Verification items for the finished model (mm, model axes). Face numbers are marked on the shaded views. A direction names the side the tool comes from. Round coordinates to 2 decimals unless told otherwise and drop trailing zeros. Write each loop counter-clockwise with the first axis right and the second up, starting at its lowest first coordinate (ties: lowest second). Pieces come first, ordered by that corner, then holes. Notation, with made-up numbers: (23, -27.5) - (62, -27.5) arc R26 ccw to (62, -13.5) - close; hole circle Ø2 at (60.5, 74.25). An arc over 180 degrees is marked (long way). Answer as a JSON object with one key per item and string values.
Autodesk Inventor part; units mm, degrees
ref_plane "YZ Plane" through (0, 0, 0) normal (1, 0, 0) x (0, 1, 0)
ref_plane "XZ Plane" through (0, 0, 0) normal (0, 1, 0) x (-1, 0, 0)
ref_plane "XY Plane" through (0, 0, 0) normal (0, 0, 1) x (1, 0, 0)
sketch "Skizze1" plane through (0, 0, 0) normal (0, 0, 1) x (1, 0, 0)
  line L0 (0, 0) -> (12, 0)
  line L1 (12, 0) -> (12, 12)
  line L2 (12, 12) -> (0, 12)
  line L3 (0, 12) -> (0, 0)
  dimension "d0" = 12
  dimension "d1" = 12
extrude "Extrusion1" add sketch "Skizze1" along normal blind 5
sketch "Skizze2" plane through (0, 0, 5) normal (0, 0, 1) x (1, 0, 0)
  circle A0 centre (6, 6) radius 1
  line L0 (12, 0) -> (12, 12)
  line L1 (0, 0) -> (12, 0)
  dimension "d4" = 6
  dimension "d5" = 6
  dimension "d6" = 2
extrude "Extrusion2" add sketch "Skizze2" along normal blind 3
chamfer "Fase1" distance 0.5 angle 45 1 edges at (5, 6, 8)
sketch "Skizze3" plane through (0, 12, 0) normal (0, 1, 0) x (1, 0, 0)
  line L0 (0, 0) -> (12, 0)
  circle A0 centre (6, 0) radius 2.25
  dimension "d12" = 4.5
extrude "Extrusion3" cut sketch "Skizze3" against normal blind 4
sketch "Skizze4" plane through (0, 0, 0) normal (0, 0, -1) x (-1, 0, 0)
  circle A0 centre (-6, 6) radius 0.5
  circle A1 centre (-6, 6) radius 5.4
  point P0 (0, 0)
ref_plane "Arbeitsebene1" through (0, 0, 0.5) normal (0, 0, -1) x (-1, 0, 0)
sketch "Skizze5" plane through (0, 0, 0.5) normal (0, 0, -1) x (-1, 0, 0)
  circle A0 centre (-6, 6) radius 0.5
  circle A1 centre (-6, 6) radius 3.55
  point P0 (0, 0)
  dimension "d18" = 7.1
extrude "Extrusion5" cut sketch "Skizze5" against normal blind 2.7
sketch "Skizze6" plane through (0, 12, 5) normal (0, 1, 0) x (1, 0, 0)
  line L0 (12, 4.5) -> (0, 4.5)
  line L1 (0, 4.5) -> (0, 5)
  line L2 (0, 5) -> (12, 5)
  line L3 (12, 5) -> (12, 4.5)
  line L4 (0, 5) -> (0, 0)
  line L5 (3.75, 5) -> (0, 5)
  line L6 (12, 5) -> (12, 0)
  line L7 (3.8063, 4.5) -> (8.1937, 4.5)
  dimension "d24" = 0
  dimension "d25" = 0
  dimension "d26" = 0
  dimension "d27" = 0
extrude "Extrusion6" cut sketch "Skizze6" against normal blind 20
fillet "Rundung1" radius 2 1 edges at (9.55, 6, 3.2)
properties part number "Elektrodenhaltr3.0"
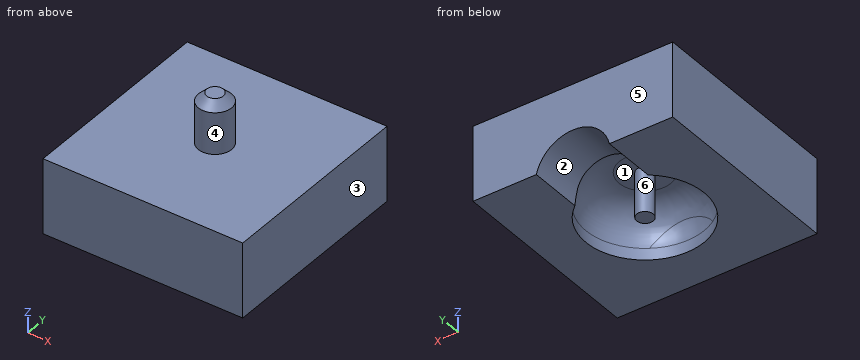
Q1. Gauge pin test, flat ends, axial feed: P1, Ø1, axis at x = 5.5, z = 3.5, coming from the -Y side; P2, Ø1, axis at x = 9.5, y = 10.5, coming from the +Z side. Record the tip position at first contact, or that the pin passes through.
Geometry check:
{"P1": "stops at y = 0", "P2": "stops at z = 5"}
Q2. Section check A-A, the plane x = 10.75. Record the cut outline in (y, z).
Geometry check:
{"outline": "(0, 0.5) - (12, 0.5) - (12, 5) - (0, 5) - close"}
Q3. Set-up check for the marked faces 1, 2 and 3: record each of +Z, -Z, +X, -X, +Y, -Y from which the full face is reachable in a straight line by a thin tool's end or side.
Geometry check:
{"face 1": "-Z", "face 2": "-Z, +Y", "face 3": "+Z, -Z, +X, +Y, -Y"}
Q4. Section check B-B, the plane y = 11. Record the cut outline in (x, z).
Geometry check:
{"outline": "(0, 0.5) - (3.81, 0.5) arc R2.25 cw to (8.19, 0.5) - (12, 0.5) - (12, 5) - (0, 5) - close"}
Q5. Release check for a two-part mould opening along X. For the marked faces 4, 5 and 6 record: released by +X, released by -X, zero draft, split by the parting line, or undercut.
Geometry check:
{"face 4": "split by the parting line", "face 5": "zero draft", "face 6": "undercut"}
Q6. Material ranges on line 1 along Y through (x, z) = (6, 1); line 2 along Z through (x, y) = (1.5, 7.5); line 3 along Y through (x, z) = (5.75, 7), recorded low to high. Write a range as [from, to].
Geometry check:
{"line 1": "y = [0, 2.45], [5.5, 6.5]", "line 2": "z = [0.5, 5]", "line 3": "y = [5.03, 6.97]"}
